Could you check a few things on this model? Use its own coordinates, in mm. A direction names the side the tool comes from. Give positions to 0.01 mm unless a question says otherwise; leave off trailing zeros. Order: outer loops, then holes, each group sorted by start corner. A loop starts at its lowest first (then second) coordinate and runs counter-clockwise, first axis right, second up.
(1) If I drill on probe 1 along Y at (x, z) = (8.5, 0.85); probe 2 along Y at (x, z) = (4, 1.25); probe 3 along X at (y, z) = (25.5, 1.2), over which ranges is the centre line in solid material (lowest first)?
(2) Imagine slicing it at D-D, the plane z = 0.8. State how many separate pieces and enclosed holes the cut face has, then the cut area to 3 significant figures.
(3) On a 3-axis mill with a long thin cutter (end or side, diameter ignored), from which of +Z, -Z, +X, -X, +Y, -Y can I reach the whole of each face in a straight line? I mean faces 4 (the flat face through (46, 7.619, 1)), 5 (the flat face through (28, 35, 1)). Say none if no direction works.
(4) If we mould it in two halves opening along X, with no side actions, what happens to faces 1 (the flat face through (41.146, 11.61, 0.986)), 2 (the cylindrical face through (0.86, 0.9, 0.99)), 3 (the flat face through (55, 17, 1))? For each: released by +X, released by -X, zero draft, split by the parting line, or undercut.
(5) Imagine slicing it at B-B, the plane x = 4. Write out the boundary of the cut face in (y, z), then the cut area to 3 significant figures.
(6) Will this pin go through, and if not, where does the flat tip stop? pin 1 (2 mm diameter, centred on x = 5.5, y = 21.5, fed in from -Z).
(7) Imagine slicing it at C-C, the plane y = 26. Write out the boundary of the cut face in (x, z).
(8) Imagine slicing it at A-A, the plane y = 31. Write out the boundary of the cut face in (x, z), then the cut area to 3 significant figures.
from build123d import *

# Parameters (mm, degrees)
F0_R     = 1.5
F1_DEPTH = 2


with BuildPart() as f1:
    # F0 (on Top) → F1 (new body)
    with BuildSketch(Plane.XY):
        with BuildLine():
            ThreePointArc((0, 3), (0.8786796564, 0.8786796564), (3, 0))
            Line((3, 0), (52, 0))
            ThreePointArc((52, 0), (54.1213203436, 0.8786796564), (55, 3))
            Line((55, 3), (55, 32))
            ThreePointArc((55, 32), (54.1213203436, 34.1213203436), (52, 35))
            Line((52, 35), (3, 35))
            ThreePointArc((3, 35), (0.8786796564, 34.1213203436), (0, 32))
            Line((0, 32), (0, 3))
        make_face()
        with BuildLine():
            Line((19.287783905, 7.6187494158), (15.552855407, 7.6187494158))
            Line((15.552855407, 7.6187494158), (10.9262547902, 22.6930554257))
            Line((10.9262547902, 22.6930554257), (10.8084867745, 22.6930554257))
            add(Edge.make_bspline(
                [(10.8084867745, 22.6930554257), (11.0608468081, 18.0958968128), (11.0608468081, 16.5565006075)],
                knots=[0, 0, 0, 1, 1, 1], degree=2))
            Line((11.0608468081, 16.5565006075), (11.0608468081, 7.6187494158))
            Line((11.0608468081, 7.6187494158), (7.4184503225, 7.6187494158))
            Line((7.4184503225, 7.6187494158), (7.4184503225, 26.8359659781))
            Line((7.4184503225, 26.8359659781), (12.9661650622, 26.8359659781))
            Line((12.9661650622, 26.8359659781), (17.5128516684, 12.1402000187))
            Line((17.5128516684, 12.1402000187), (17.592765679, 12.1402000187))
            Line((17.592765679, 12.1402000187), (22.4170483223, 26.8359659781))
            Line((22.4170483223, 26.8359659781), (27.9605570614, 26.8359659781))
            Line((27.9605570614, 26.8359659781), (27.9605570614, 7.6187494158))
            Line((27.9605570614, 7.6187494158), (24.162538555, 7.6187494158))
            Line((24.162538555, 7.6187494158), (24.162538555, 16.7163286288))
            add(Edge.make_bspline(
                [(24.162538555, 16.7163286288), (24.162538555, 17.3598467146), (24.1835685578, 18.2010468268)],
                knots=[0, 0, 0, 1, 1, 1], degree=2))
            add(Edge.make_bspline(
                [(24.1835685578, 18.2010468268), (24.2045985606, 19.042246939), (24.3602205814, 22.6678194224)],
                knots=[0, 0, 0, 1, 1, 1], degree=2))
            Line((24.3602205814, 22.6678194224), (24.2424525657, 22.6678194224))
            Line((24.2424525657, 22.6678194224), (19.287783905, 7.6187494158))
        make_face(mode=Mode.SUBTRACT)
        Polygon((41.4996728666, 18.3314328442), (48.2545097673, 7.6187494158), (43.6279091504, 7.6187494158), (38.5933264791, 15.7153004954), (36.8730722497, 14.4787363305), (36.8730722497, 7.6187494158), (32.7974577063, 7.6187494158), (32.7974577063, 26.8359659781), (36.8730722497, 26.8359659781), (36.8730722497, 18.0412188055), (38.4755584634, 20.3040471072), (43.6825871577, 26.8359659781), (48.2040377605, 26.8359659781), align=None, mode=Mode.SUBTRACT)
        with Locations((4, 31)):
            Circle(F0_R, mode=Mode.SUBTRACT)
    extrude(amount=F1_DEPTH)


solid = f1.part
Answer block:
1. probe 1: y = 0 to 7.62, 26.84 to 35
1. probe 2: y = 0 to 29.5, 32.5 to 35
1. probe 3: x = 0 to 7.42, 13.38 to 21.98, 27.96 to 32.8, 36.87 to 42.62, 47.15 to 55
2. separate pieces: 1
2. enclosed holes: 3
2. area: 1,490 mm2
3. face 4: +Z, -Z
3. face 5: +Z, -Z, +X, -X, +Y
4. face 1: undercut
4. face 2: released by -X
4. face 3: released by +X
5. outline: (0, 0) - (29.5, 0) - (29.5, 2) - (0, 2) - close; (32.5, 0) - (35, 0) - (35, 2) - (32.5, 2) - close
5. area: 64.0 mm2
6. pin 1: stops at z = 0
7. outline: (0, 0) - (7.42, 0) - (7.42, 2) - (0, 2) - close; (13.22, 0) - (22.14, 0) - (22.14, 2) - (13.22, 2) - close; (27.96, 0) - (32.8, 0) - (32.8, 2) - (27.96, 2) - close; (36.87, 0) - (43.02, 0) - (43.02, 2) - (36.87, 2) - close; (47.55, 0) - (55, 0) - (55, 2) - (47.55, 2) - close
8. outline: (0, 0) - (2.5, 0) - (2.5, 2) - (0, 2) - close; (5.5, 0) - (55, 0) - (55, 2) - (5.5, 2) - close
8. area: 104 mm2
